Model file for the job. Use its own axes, mm. A direction names the side the tool comes from. Coordinates: 2 decimals unless noted, no trailing zeros. Order: outer loops, then holes, each group sorted by start corner. A loop starts at its lowest first (then second) coordinate and runs counter-clockwise, first axis right, second up.
from build123d import *

# Parameters (mm, degrees)
F1_DEPTH = 50
F2_DEPTH = 3
F3_R     = 3
F4_R     = 3
F6_D     = 3.3
F7_R     = 1
F8_R     = 1


with BuildPart() as f1:
    # F0 (on Top) → F1 (new body)
    with BuildSketch(Plane.XY):
        Polygon((-155, 0), (0, 0), (0, 3), (-142, 3), (-152, 3), (-152, 13), (-152, 53), (-155, 53), (-155, 3), align=None)
    extrude(amount=F1_DEPTH)

    # F0 (on Top) → F2 (join)
    with BuildSketch(Plane.XY):
        Polygon((-152, 3), (-142, 3), (-152, 13), align=None)
    extrude(amount=F2_DEPTH)

    # F3
    f3_edges = [f1.edges().sort_by_distance(p)[0] for p in [
        (-152, 3, 26.5),
    ]]
    fillet(f3_edges, radius=F3_R)

    # F4
    f4_edges = [f1.edges().sort_by_distance(p)[0] for p in [
        (-155, 0, 25),
    ]]
    fillet(f4_edges, radius=F4_R)

    # F6 (through all)
    with Locations(Plane.XZ):
        with Locations((-30, 30), (-67.5, 30)):
            Hole(F6_D / 2)

    # F7
    f7_edges = [f1.edges().sort_by_distance(p)[0] for p in [
        (-76, 0, 50),
        (-74.5, 3, 50),
        (-155, 28, 50),
        (-152, 29.5, 50),
        (-151.12132, 3.87868, 50),
        (-154.12132, 0.87868, 50),
    ]]
    fillet(f7_edges, radius=F7_R)

    # F8
    f8_edges = [f1.edges().sort_by_distance(p)[0] for p in [
        (-152, 53, 24.5),
        (-155, 53, 24.5),
        (-152.292893, 53, 49.707107),
        (-153.5, 53, 0),
        (-153.5, 53, 50),
        (-154.707107, 53, 49.707107),
    ]]
    fillet(f8_edges, radius=F8_R)


solid = f1.part
Q1. Cut at C-C, the plane z = 37.5. List the corners of the cut face in (x, y).
Established:
outline: (-155, 3) arc R3 ccw to (-152, 0) - (0, 0) - (0, 3) - (-149, 3) arc R3 cw to (-152, 6) - (-152, 52) arc R1 ccw to (-153, 53) - (-154, 53) arc R1 ccw to (-155, 52) - close
Q2. Drop flat-ended pins along their axis: P1, Ø5, axis at x = -68.5, z = 37, coming from the +Y side; P2, Ø14, axis at y = 30, z = 18, coming from the +X side; P3, Ø5, axis at x = -148, y = 6.5, coming from the +Z side. Give the stop position or say it passes through.
Established:
P1: stops at y = 3
P2: stops at x = -152
P3: stops at z = 3
Q3. Cut at D-D, the plane y = 25. List the corners of the cut face in (x, z), plus the area to 3 significant figures.
Established:
outline: (-155, 0) - (-152, 0) - (-152, 49) arc R1 ccw to (-153, 50) - (-154, 50) arc R1 ccw to (-155, 49) - close
area: 150 mm2
Q4. Probe line 1 (Z direction, x = -30, y = 2.1); line 2 (Y direction, x = -86, z = 4.5); line 3 (X direction, y = 18.5, z = 9). List the from-to ranges inside material, lowest first.
Established:
line 1: z = 0 to 28.35, 31.65 to 49.99
line 2: y = 0 to 3
line 3: x = -155 to -152
Q5. Which spindle directions (+Z, -Z, +X, -X, +Y, -Y) get a long thin tool onto all of the face, cutting with end or side? Do faces 1 (the face through (-154.1, 0.86, 24.84)), 2 (the face through (-151.1, 3.86, 26.32)). Say none if no direction does.
Established:
face 1: +Z, -Z, -X, -Y
face 2: +Z, +X, +Y
Q6. Mould opens along X. For faces 3 (the face through (0, 1, 25)), 4 (the face through (-77, 0, 24)), 5 (the face through (-66.284, 1.521, 31.115)) say: pulls with the +X half, pulls with the -X half, needs draft (parallel to the pull), parting line crosses it, or undercut.
Established:
face 3: pulls with the +X half
face 4: needs draft
face 5: undercut
Q7. Cut at B-B, the plane z = 30. List the corners of the cut face in (x, y).
Established:
outline: (-155, 3) arc R3 ccw to (-152, 0) - (-69.15, 0) - (-69.15, 3) - (-149, 3) arc R3 cw to (-152, 6) - (-152, 52) arc R1 ccw to (-153, 53) - (-154, 53) arc R1 ccw to (-155, 52) - close; (-65.85, 0) - (-31.65, 0) - (-31.65, 3) - (-65.85, 3) - close; (-28.35, 0) - (0, 0) - (0, 3) - (-28.35, 3) - close
Q8. Cut at A-A, the plane x = -30. List the corners of the cut face in (y, z).
Established:
outline: (0, 0) - (3, 0) - (3, 28.35) - (0, 28.35) - close; (0, 31.65) - (3, 31.65) - (3, 49) arc R1 ccw to (2, 50) - (1, 50) arc R1 ccw to (0, 49) - close
